Input: part model. Units: mm. Frame: model coordinates. Give positions to 0.01 mm unless a question says otherwise; leave off trailing zeros. Loops run counter-clockwise (first coordinate to the right, second up) from the corner with the lowest first, then second, coordinate; pieces in that order, holes last. Notation, with made-up numbers: (33, -2.75) - (47, -2.75) arc R20 cw to (47, 20.25) - close; hole circle Ø4 at (20.5, 28). An arc over 180 degrees is marked (long way). Answer as a JSON object with one key per item and string values. Group by question number.
(1) Pin query (flat end, axial travel): P1, Ø0.9, axis at x = -5, z = 2, coming from the +Y side; P2, Ø1.5, axis at x = -5, z = 2, coming from the -Y side; P3, Ø1.5, axis at y = -8.5, z = 1, coming from the +X side. Return the tip coordinate at first contact, or that it passes through.
(2) Section query D-D (y = 62.5). Return loops of the section in (x, z).
(3) Material intervals for L1, parallel to X at y = 17, z = 1.7; L2, parallel to Y at x = 13.75, z = 1.6; L3, parallel to X at y = 70, z = 1.2, sorted ascending.
(4) Section query A-A (y = -40). Return loops of the section in (x, z).
(5) Section query C-C (z = 1). Count the separate pieces of the cut face and the enclosed holes in it, plus the area to 3 significant figures.
(6) Section query B-B (x = -55). Return loops of the section in (y, z).
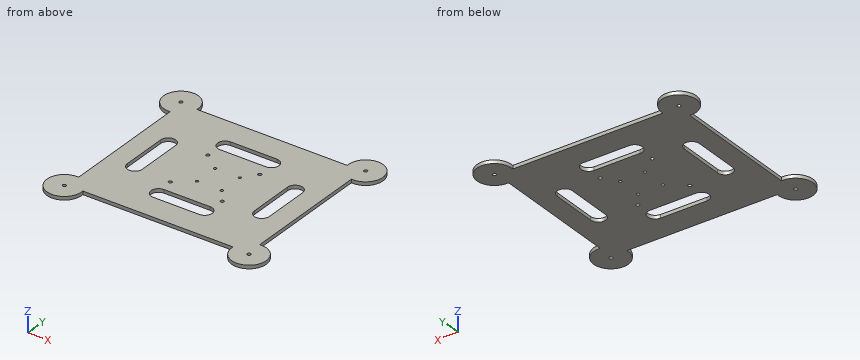
Autodesk Inventor part; units mm, degrees
ref_plane "YZ Plane" through (0, 0, 0) normal (1, 0, 0) x (0, 1, 0)
ref_plane "XZ Plane" through (0, 0, 0) normal (0, 1, 0) x (-1, 0, 0)
ref_plane "XY Plane" through (0, 0, 0) normal (0, 0, 1) x (1, 0, 0)
sketch "Sketch1" plane through (0, 0, 0) normal (0, 0, 1) x (1, 0, 0)
  point P0 (0, 0)
sketch "Sketch2" plane through (0, 0, 0) normal (0, 0, 1) x (1, 0, 0)
  line L0 (78.4999, -68.5) -> (-78.4999, -68.5)
  line L1 (-78.4999, -68.5) -> (-78.4999, 68.5)
  line L2 (-78.4999, 68.5) -> (78.4999, 68.5)
  line L3 (78.4999, 68.5) -> (78.4999, -68.5)
  circle A0 centre (80, 70) radius 14.9999
  circle A1 centre (-80, 70) radius 14.9999
  circle A2 centre (-80, -70) radius 14.9999
  circle A3 centre (80, -70) radius 14.9999
  point P0 (78.4999, -55.0753)
  point P1 (78.4999, 55.0753)
  point P2 (65.0752, 68.5)
  point P3 (-65.0752, 68.5)
  point P4 (-78.4999, 55.0753)
  point P5 (-78.4999, -55.0753)
  point P6 (-65.0752, -68.5)
  point P7 (65.0752, -68.5)
extrude "Extrusion1" add sketch "Sketch2" along normal blind 3
sketch "Sketch5" plane through (0, 0, 3) normal (0, 0, 1) x (1, 0, 0)
  circle A0 centre (80, 70) radius 1.4999
  circle A1 centre (-80, 70) radius 1.4999
  circle A2 centre (-80, -70) radius 1.4999
  circle A3 centre (80, -70) radius 1.4999
extrude "Extrusion2" cut sketch "Sketch5" against normal blind 10
sketch "Sketch6" plane through (0, 0, 3) normal (0, 0, 1) x (1, 0, 0)
  point P0 (0, 0)
sketch "Cable cutouts" plane through (0, 0, 3) normal (0, 0, 1) x (1, 0, 0)
  line L0 (65.0752, 68.5) -> (-65.0752, 68.5)
  line L1 (-20.0003, 40) -> (20.0003, 40) construction
  line L2 (-20.0003, 33.4981) -> (20.0003, 33.4981)
  line L3 (20.0003, 46.5019) -> (-20.0003, 46.5019)
  arc A0 (-20.0003, 46.5019) -> (-20.0003, 33.4981) centre (-20.0003, 40) ccw
  arc A1 (20.0003, 33.4981) -> (20.0003, 46.5019) centre (20.0003, 40) ccw
  line L4 (-20.0003, -40) -> (20.0003, -40) construction
  line L5 (-20.0003, -46.5019) -> (20.0003, -46.5019)
  line L6 (20.0003, -33.4981) -> (-20.0003, -33.4981)
  arc A2 (-20.0003, -33.4981) -> (-20.0003, -46.5019) centre (-20.0003, -40) ccw
  arc A3 (20.0003, -46.5019) -> (20.0003, -33.4981) centre (20.0003, -40) ccw
  line L7 (55, -20.0003) -> (55, 20.0003) construction
  arc A4 (48.4981, -20.0003) -> (61.5019, -20.0003) centre (55, -20.0003) ccw
  arc A5 (61.5019, 20.0003) -> (48.4981, 20.0003) centre (55, 20.0003) ccw
  line L8 (48.4981, 20.0003) -> (48.4981, -20.0003)
  line L9 (61.5019, -20.0003) -> (61.5019, 20.0003)
  line L10 (-55, -20.0003) -> (-55, 20.0003) construction
  arc A6 (-61.5019, -20.0003) -> (-48.4981, -20.0003) centre (-55, -20.0003) ccw
  arc A7 (-48.4981, 20.0003) -> (-61.5019, 20.0003) centre (-55, 20.0003) ccw
  line L11 (-61.5019, 20.0003) -> (-61.5019, -20.0003)
  line L12 (-48.4981, -20.0003) -> (-48.4981, 20.0003)
extrude "Extrusion4" cut sketch "Cable cutouts" against normal blind 10
sketch "Pixhawk 3 Pro mount holes" plane through (0, 0, 3) normal (0, 0, 1) x (1, 0, 0)
  circle A0 centre (13.75, 10.75) radius 1.2498
  circle A1 centre (-7.75, 10.75) radius 1.2498
  circle A2 centre (-7.75, -10.75) radius 1.2498
  circle A3 centre (13.75, -10.75) radius 1.2498
extrude "Extrusion5" cut sketch "Pixhawk 3 Pro mount holes" against normal blind 10
sketch "Anti-vibration mount holes" plane through (0, 0, 3) normal (0, 0, 1) x (1, 0, 0)
  circle A0 centre (22.5, 22.5) radius 1.4999
  circle A1 centre (-22.5, 22.5) radius 1.4999
  circle A2 centre (-22.5, -22.5) radius 1.4999
  circle A3 centre (22.5, -22.5) radius 1.4999
extrude "Extrusion7" cut sketch "Anti-vibration mount holes" against normal blind 10
properties part number "Payload bay KPM" material "CFRP"
Recorded:
{
 "1": {"P1": "stops at y = 68.5", "P2": "stops at y = -68.5", "P3": "stops at x = 78.5"},
 "2": {"outline": "(-92.99, 0) - (92.99, 0) - (92.99, 3) - (-92.99, 3) - close"},
 "3": {"L1": "x = -78.5 to -61.5, -48.5 to 48.5, 61.5 to 78.5", "L2": "y = -68.5 to -46.5, -33.5 to -12, -9.5 to 9.5, 12 to 33.5, 46.5 to 68.5", "L3": "x = -95 to -81.5, -78.5 to -65, 65 to 78.5, 81.5 to 95"},
 "4": {"outline": "(-78.5, 0) - (-26.5, 0) - (-26.5, 3) - (-78.5, 3) - close; (26.5, 0) - (78.5, 0) - (78.5, 3) - (26.5, 3) - close"},
 "5": {"separate pieces": "1", "enclosed holes": "16", "area": "21,100 mm^2"},
 "6": {"outline": "(-68.5, 0) - (-26.5, 0) - (-26.5, 3) - (-68.5, 3) - close; (26.5, 0) - (68.5, 0) - (68.5, 3) - (26.5, 3) - close"}
}
